The model under review builds one solid part; all positions refer to its coordinate system, in mm. A direction names the side the tool comes from. Coordinates: 2 decimals unless noted, no trailing zeros. Loops run counter-clockwise (first coordinate to the right, second up) from the corner with the lowest first, then second, coordinate; pieces in that order, holes last. Notation, with made-up numbers: M 39,84 L 56,84 A31 ccw 56,121 Z; hole C 28.5,3.25 d4. An arc over 180 degrees is marked long. One line per item, written item: value.
Autodesk Inventor part; units mm, degrees
ref_plane "YZ Plane" through (0, 0, 0) normal (1, 0, 0) x (0, 1, 0)
ref_plane "XZ Plane" through (0, 0, 0) normal (0, 1, 0) x (-1, 0, 0)
ref_plane "XY Plane" through (0, 0, 0) normal (0, 0, 1) x (1, 0, 0)
sketch "Sketch1" plane through (0, 0, 0) normal (0, 0, 1) x (1, 0, 0)
  line L0 (-5.0907, -72.0223) -> (-5.0907, -92.0223)
  line L1 (-5.0907, -92.0223) -> (-25.0907, -92.0223)
  line L2 (-25.0907, -92.0223) -> (-25.0907, -72.0223)
  line L3 (-25.0907, -72.0223) -> (-5.0907, -72.0223)
  line L4 (-5.0907, 0) -> (-25.0907, 0)
  line L5 (-25.0907, 0) -> (-25.0907, 20)
  line L6 (-25.0907, 20) -> (-5.0907, 20)
  line L7 (-5.0907, 20) -> (-5.0907, 0)
  line L8 (-22.7107, -2.7) -> (-2.3907, -2.7)
  line L9 (-2.3907, -2.7) -> (-2.3907, 22.7)
  line L10 (-2.3907, 22.7) -> (-27.7907, 22.7)
  line L11 (-27.7907, 22.7) -> (-27.7907, -94.7223)
  line L12 (-27.7907, -94.7223) -> (-2.3907, -94.7223)
  line L13 (-2.3907, -94.7223) -> (-2.3907, -69.3223)
  line L14 (-2.3907, -69.3223) -> (-22.7107, -69.3223)
  line L15 (-22.7107, -2.7) -> (-22.7107, -69.3223)
  line L16 (-25.0907, 20) -> (-25.0907, 22.7)
  line L17 (-22.7107, -2.7) -> (-22.7107, 0)
  line L18 (-22.7107, -69.3223) -> (-22.7107, -72.0223)
  line L19 (-25.0907, -92.0223) -> (-27.7907, -92.0223)
  line L20 (-25.0907, 20) -> (-27.7907, 20)
  line L21 (-5.0907, 0) -> (-5.0907, -2.7)
  line L22 (-5.0907, -72.0223) -> (-5.0907, -69.3223)
  point P0 (0, 0)
extrude "Extrusion1" add sketch "Sketch1" against normal blind 50 contours L3 L18 L14 L22 | L3 L2 L19 L11 L20 L5 L4 L17 L15 L18 | L17 L4 L21 L8
sketch "Sketch2" plane through (-27.7907, -92.0223, 0) normal (-1, 0, 0) x (0, 0, 1)
  line L0 (0, 112.0223) -> (0, 0)
  line L1 (0, 112.0223) -> (-50, 112.0223)
  line L2 (-50, 0) -> (-50, 112.0223)
  line L3 (0, 0) -> (-50, 0)
  circle A0 centre (-25, 56.0111) radius 12.5
  line L4 (-25, 56.0111) -> (-40.5, 56.0111)
  line L5 (-40.5, 56.0111) -> (-40.5, 71.5111)
  circle A1 centre (-40.5, 71.5111) radius 2
  circle A2 centre (-40.5, 40.5111) radius 2
  circle A3 centre (-9.5, 71.5111) radius 2
  circle A4 centre (-9.5, 40.5111) radius 2
  point P0 (0, 92.0223)
  dimension "d2" = 25
  dimension "d3" = 15.5
  dimension "d4" = 15.5
  dimension "d5" = 4
  dimension "d8" = 31
  dimension "d11" = 31
extrude "Extrusion2" cut sketch "Sketch2" against normal blind 50 contours A0 | A1 | A2 | A3 | A4
sketch "Sketch3" plane through (-27.7907, -92.0223, 0) normal (-1, 0, 0) x (0, 0, 1)
  circle A0 centre (-9.5, 40.5111) radius 2
  circle A1 centre (-40.5, 40.5111) radius 2
  circle A2 centre (-40.5, 71.5111) radius 2
  circle A3 centre (-9.5, 71.5111) radius 2
  circle A4 centre (-25, 56.0111) radius 12.5
  line L0 (0, 112.0223) -> (0, 0)
  line L1 (0, 112.0223) -> (-50, 112.0223)
  line L2 (-50, 0) -> (-50, 112.0223)
  line L3 (0, 0) -> (-50, 0)
  line L4 (-619.5788, 92.0223) -> (142.4212, 92.0223)
  line L5 (142.4212, 112.0223) -> (142.4212, 92.0223)
  line L6 (142.4212, 112.0223) -> (-619.5788, 112.0223)
  line L7 (-619.5788, 92.0223) -> (-619.5788, 112.0223)
  circle A5 centre (-25, 102.0223) radius 2
  circle A6 centre (-9.5, 40.5111) radius 2
  circle A7 centre (-40.5, 40.5111) radius 2
  circle A8 centre (-40.5, 71.5111) radius 2
  circle A9 centre (-9.5, 71.5111) radius 2
  circle A10 centre (-25, 56.0111) radius 12.5
  line L8 (0, 112.0223) -> (0, 0)
  line L9 (0, 112.0223) -> (-50, 112.0223)
  line L10 (-50, 0) -> (-50, 112.0223)
  line L11 (0, 0) -> (-50, 0)
  line L12 (-619.5855, 0) -> (142.4145, 0)
  line L13 (142.4145, 20) -> (142.4145, 0)
  line L14 (142.4145, 20) -> (-619.5855, 20)
  line L15 (-619.5855, 0) -> (-619.5855, 20)
  circle A11 centre (-25, 10) radius 2
  point P0 (0, 92.0223)
  dimension "d16" = 4
  dimension "d17" = 4
extrude "Extrusion3" cut sketch "Sketch3" against normal blind 50 contours A5 | A11
properties part number "SecondExtruder"
(1) Add section D-D on z = -9.5. State the section outline as (x, y) points, then the cut area to 3 significant figures.
Checks:
outline: M -27.79,-92.02 L -25.09,-92.02 L -25.09,-72.02 L -5.09,-72.02 L -5.09,-69.32 L -22.71,-69.32 L -22.71,-53.51 L -27.79,-53.51 Z; M -27.79,-49.51 L -22.71,-49.51 L -22.71,-22.51 L -27.79,-22.51 Z; M -27.79,-18.51 L -22.71,-18.51 L -22.71,-2.7 L -5.09,-2.7 L -5.09,0 L -25.09,0 L -25.09,20 L -27.79,20 Z
area: 528 mm^2
(2) Add section A-A on y = 10. State the section outline as (x, z) points.
Checks:
outline: M -27.79,-50 L -25.09,-50 L -25.09,-27 L -27.79,-27 Z; M -27.79,-23 L -25.09,-23 L -25.09,0 L -27.79,0 Z
(3) Add section B-B on z = -25. State the section outline as (x, y) points.
Checks:
outline: M -27.79,-92.02 L -25.09,-92.02 L -25.09,-84.02 L -27.79,-84.02 Z; M -27.79,-80.02 L -25.09,-80.02 L -25.09,-72.02 L -5.09,-72.02 L -5.09,-69.32 L -22.71,-69.32 L -22.71,-48.51 L -27.79,-48.51 Z; M -27.79,-23.51 L -22.71,-23.51 L -22.71,-2.7 L -5.09,-2.7 L -5.09,0 L -25.09,0 L -25.09,8 L -27.79,8 Z; M -27.79,12 L -25.09,12 L -25.09,20 L -27.79,20 Z
(4) Insertion check: pin 1 Ø3 at (y, z) = (-74, -30) entering from +X; pin 2 Ø6 at (x, z) = (-16.5, -34.5) entering from +Y; pin 3 Ø6.5 at (y, z) = (-20.51, -40.5) entering from +X. Each pin has a flat end and moves straight along its axis. Give the tip position at first contact, or say it passes through.
Checks:
pin 1: x = -25.09
pin 2: y = 0
pin 3: x = -22.71
(5) Draft analysis for pull direction Y (two halves, no side actions). For faces 6 (the face through (-25.286, -53.286, -39.577)), 7 (the face through (-26, -92.022, -25)), 8 (the face through (-25.286, -43.617, -34.92)), 9 (the face through (-27.791, -23, -25)), state which applies: pulls with the +Y half, pulls with the -Y half, needs draft (parallel to the pull), parting line crosses it, or undercut.
Checks:
face 6: undercut
face 7: pulls with the -Y half
face 8: undercut
face 9: needs draft
(6) Add section C-C on x = -17.5. State the section outline as (y, z) points.
Checks:
outline: M -72.02,-50 L -69.32,-50 L -69.32,0 L -72.02,0 Z; M -2.7,-50 L 0,-50 L 0,0 L -2.7,0 Z
(7) To check wall thickness, follow L1, parallel to Y at x = -26.1, z = -9.5; L2, parallel to Y at x = -26.2, z = -25; L3, parallel to Y at x = -24.9, z = -9.5. State the ranges of each line that lie inside material, in increasing order. Write a range as [from, to].
Checks:
L1: [-92.02, -53.51], [-49.51, -22.51], [-18.51, 20]
L2: [-92.02, -84.02], [-80.02, -48.51], [-23.51, 8], [12, 20]
L3: [-72.02, -53.51], [-49.51, -22.51], [-18.51, 0]
(8) Tool access review of faces 1 (the face through (-26.46, -83.975, -25.434)), 2 (the face through (-24, -32, -50)), 3 (the face through (-14, -69.322, -25)), 4 (the face through (-15, -72.022, -25)), 5 (the face through (-25.091, 7.6, -24.6)): name each direction out of +Z, -Z, +X, -X, +Y, -Y from which nothing blocks a thin tool from reaching the whole face with its end or side.
Checks:
face 1: +X, -X
face 2: -Z, +X, -X, +Y, -Y
face 3: +Z, -Z, +X
face 4: +Z, -Z, +X, -Y
face 5: +Z, -Z, +X, +Y
